Geometry: final body of the model. Coordinates: model frame, mm. Face numbers are marked on the shaded views. A direction names the side the tool comes from. Round coordinates to 2 decimals unless told otherwise and drop trailing zeros. Loops run counter-clockwise (first coordinate to the right, second up) from the corner with the lowest first, then second, coordinate; pieces in that order, holes last. Notation, with made-up numbers: M -12,31.5 L 3,31.5 A23 ccw 3,63.5 Z; hole C 82.5,22 d11. An arc over 180 degrees is marked long. Return JSON: item names as keys, results as strings.
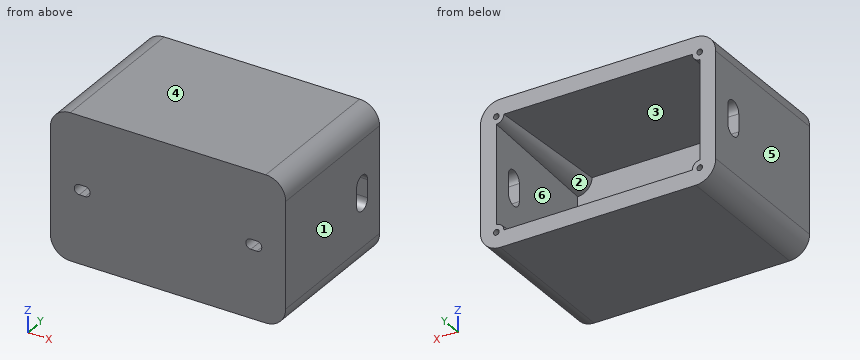
from build123d import *

# Parameters (mm, degrees)
SKETCH1_W                     = 118
SKETCH1_H                     = 73
BOSS_EXTRUDE1_DEPTH           = 75
SKETCH3_W                     = 102
SKETCH3_H                     = 57
CUT_EXTRUDE2_DEPTH            = 65
FILLET1_R                     = 10
CUT_EXTRUDE3_DEPTH            = 103.167754208
SKETCH5_R                     = 7.171572875
BOSS_EXTRUDE2_DEPTH           = 65
BOSS_EXTRUDE2_DRAFT           = 3
BOSS_EXTRUDE2_PROFILE_2_DEPTH = 65
BOSS_EXTRUDE2_PROFILE_2_DRAFT = 3
BOSS_EXTRUDE2_PROFILE_3_DEPTH = 65
BOSS_EXTRUDE2_PROFILE_3_DRAFT = 3
BOSS_EXTRUDE2_PROFILE_4_DEPTH = 65
BOSS_EXTRUDE2_PROFILE_4_DRAFT = 3
SKETCH9_R                     = 1.4
CUT_EXTRUDE6_DEPTH            = 5
CUT_EXTRUDE7_DEPTH            = 10000


with BuildPart() as part:
    # Sketch1 → Boss-Extrude1 (new body)
    with BuildSketch(Plane(origin=(0, 0, 0), x_dir=(1, 0, 0), z_dir=(0, 1, 0))):
        Rectangle(SKETCH1_W, SKETCH1_H)
    extrude(amount=BOSS_EXTRUDE1_DEPTH)

    # Sketch3 → Cut-Extrude2 (cut)
    with BuildSketch(Plane(origin=(0, 75, 0), x_dir=(1, 0, 0), z_dir=(0, 1, 0))):
        Rectangle(SKETCH3_W, SKETCH3_H)
    extrude(amount=-CUT_EXTRUDE2_DEPTH, mode=Mode.SUBTRACT)

    # Fillet1
    fillet1_edges = [part.edges().sort_by_distance(p)[0] for p in [
        (-59, 37.5, -36.5),
        (59, 37.5, -36.5),
        (59, 37.5, 36.5),
        (-59, 37.5, 36.5),
    ]]
    fillet(fillet1_edges, radius=FILLET1_R)

    # Sketch4 → Cut-Extrude3 (cut, through all)
    with BuildSketch(Plane.XZ):
        with BuildLine():
            Line((-44.5, -2.5), (-41.5, -2.5))
            ThreePointArc((-41.5, -2.5), (-39, 0), (-41.5, 2.5))
            Line((-41.5, 2.5), (-44.5, 2.5))
            ThreePointArc((-44.5, 2.5), (-47, 0), (-44.5, -2.5))
        make_face()
        with BuildLine():
            ThreePointArc((41.5, -2.5), (39, 0), (41.5, 2.5))
            Line((41.5, 2.5), (44.5, 2.5))
            ThreePointArc((44.5, 2.5), (47, 0), (44.5, -2.5))
            Line((44.5, -2.5), (41.5, -2.5))
        make_face()
    extrude(amount=-CUT_EXTRUDE3_DEPTH, mode=Mode.SUBTRACT)


with BuildPart() as boss_extrude2_tool:
    # Sketch5 → Boss-Extrude2 (with draft: the straight prism first)
    with BuildSketch(Plane(origin=(0, 10, 0), x_dir=(1, 0, 0), z_dir=(0, 1, 0))):
        with Locations((-51, 28.5)):
            Circle(SKETCH5_R)
    extrude(amount=BOSS_EXTRUDE2_DEPTH)
    # Boss-Extrude2: the draft: its side faces are tilted about the plane it starts from
    boss_extrude2_sides = [boss_extrude2_tool.faces().sort_by_distance(p)[0] for p in [
        (-58.171572875, 42.5, -28.5),
    ]]
    draft(boss_extrude2_sides, Plane(origin=(0, 10, 0), x_dir=(1, 0, 0), z_dir=(0, 1, 0)), BOSS_EXTRUDE2_DRAFT)


with BuildPart() as part_1:
    add(part.part)

    # Boss-Extrude2: add boss_extrude2_tool
    add(boss_extrude2_tool.part)


with BuildPart() as boss_extrude2_profile_2_tool:
    # Sketch5 → Boss-Extrude2 profile 2 (with draft: the straight prism first)
    with BuildSketch(Plane(origin=(0, 10, 0), x_dir=(1, 0, 0), z_dir=(0, 1, 0))):
        with Locations((51, 28.5)):
            Circle(SKETCH5_R)
    extrude(amount=BOSS_EXTRUDE2_PROFILE_2_DEPTH)
    # Boss-Extrude2 profile 2: the draft: its side faces are tilted about the plane it starts from
    boss_extrude2_profile_2_sides = [boss_extrude2_profile_2_tool.faces().sort_by_distance(p)[0] for p in [
        (43.828427125, 42.5, -28.5),
    ]]
    draft(boss_extrude2_profile_2_sides, Plane(origin=(0, 10, 0), x_dir=(1, 0, 0), z_dir=(0, 1, 0)), BOSS_EXTRUDE2_PROFILE_2_DRAFT)


with BuildPart() as part_2:
    add(part_1.part)

    # Boss-Extrude2 profile 2: add boss_extrude2_profile_2_tool
    add(boss_extrude2_profile_2_tool.part)


with BuildPart() as boss_extrude2_profile_3_tool:
    # Sketch5 → Boss-Extrude2 profile 3 (with draft: the straight prism first)
    with BuildSketch(Plane(origin=(0, 10, 0), x_dir=(1, 0, 0), z_dir=(0, 1, 0))):
        with Locations((51, -28.5)):
            Circle(SKETCH5_R)
    extrude(amount=BOSS_EXTRUDE2_PROFILE_3_DEPTH)
    # Boss-Extrude2 profile 3: the draft: its side faces are tilted about the plane it starts from
    boss_extrude2_profile_3_sides = [boss_extrude2_profile_3_tool.faces().sort_by_distance(p)[0] for p in [
        (43.828427125, 42.5, 28.5),
    ]]
    draft(boss_extrude2_profile_3_sides, Plane(origin=(0, 10, 0), x_dir=(1, 0, 0), z_dir=(0, 1, 0)), BOSS_EXTRUDE2_PROFILE_3_DRAFT)


with BuildPart() as part_3:
    add(part_2.part)

    # Boss-Extrude2 profile 3: add boss_extrude2_profile_3_tool
    add(boss_extrude2_profile_3_tool.part)


with BuildPart() as boss_extrude2_profile_4_tool:
    # Sketch5 → Boss-Extrude2 profile 4 (with draft: the straight prism first)
    with BuildSketch(Plane(origin=(0, 10, 0), x_dir=(1, 0, 0), z_dir=(0, 1, 0))):
        with Locations((-51, -28.5)):
            Circle(SKETCH5_R)
    extrude(amount=BOSS_EXTRUDE2_PROFILE_4_DEPTH)
    # Boss-Extrude2 profile 4: the draft: its side faces are tilted about the plane it starts from
    boss_extrude2_profile_4_sides = [boss_extrude2_profile_4_tool.faces().sort_by_distance(p)[0] for p in [
        (-58.171572875, 42.5, 28.5),
    ]]
    draft(boss_extrude2_profile_4_sides, Plane(origin=(0, 10, 0), x_dir=(1, 0, 0), z_dir=(0, 1, 0)), BOSS_EXTRUDE2_PROFILE_4_DRAFT)


with BuildPart() as part_4:
    add(part_3.part)

    # Boss-Extrude2 profile 4: add boss_extrude2_profile_4_tool
    add(boss_extrude2_profile_4_tool.part)

    # Sketch9 → Cut-Extrude6 (cut)
    with BuildSketch(Plane(origin=(0, 75, 0), x_dir=(1, 0, 0), z_dir=(0, 1, 0))):
        with Locations(Location((-51, 28.5, 0), (0, 0, 270))):
            Circle(SKETCH9_R)
        with Locations(Location((51, 28.5, 0), (0, 0, 90))):
            Circle(SKETCH9_R)
        with Locations(Location((51, -28.5, 0), (0, 0, 270))):
            Circle(SKETCH9_R)
        with Locations(Location((-51, -28.5, 0), (0, 0, 90))):
            Circle(SKETCH9_R)
    extrude(amount=-CUT_EXTRUDE6_DEPTH, mode=Mode.SUBTRACT)

    # Sketch13 → Cut-Extrude7 (cut)
    with BuildSketch(Plane.ZY.offset(59)):
        with BuildLine():
            Line((-4.178843904, 65.399928421), (4.670472599, 65.399928421))
            ThreePointArc((4.670472599, 65.399928421), (9.07040102, 61), (4.670472599, 56.600071579))
            Line((4.670472599, 56.600071579), (-4.178843904, 56.600071579))
            ThreePointArc((-4.178843904, 56.600071579), (-8.578772325, 61), (-4.178843904, 65.399928421))
        make_face()
    extrude(amount=-CUT_EXTRUDE7_DEPTH, mode=Mode.SUBTRACT)


solid = part_4.part
Q1. Section query C-C (z = 16). Output: boundary loops of the cut face in (x, y), plus the area to 3 significant figures.
Determined:
{"outline": "M -59,0 L 59,0 L 59,75 L 51,75 L 51,10 L -51,10 L -51,75 L -59,75 Z", "area": "2,220 mm^2"}
Q2. Pull-direction query (X, two-part tool) for the marked faces 1, 2, 3 and 4; classes: pulls with the +X half, pulls with the -X half, needs draft (parallel to the pull), parting line crosses it, or undercut.
Determined:
{"face 1": "pulls with the +X half", "face 2": "undercut", "face 3": "undercut", "face 4": "needs draft"}
Q3. Reachability of the marked faces 5 and 6 from +Z, -Z, +X, -X, +Y, -Y: full face, straight path, thin tool, end or side. Return the list, or none.
Determined:
{"face 5": "+Z, -Z, -X, +Y, -Y", "face 6": "+Y"}
Q4. Pin query (flat end, axial travel): pin 1 (2 mm diameter, centred on x = 51, z = 28.5, fed in from +Y); pin 2 (6 mm diameter, centred on x = 7, z = -19, fed in from +Y). Return the tip coordinate at first contact, or that it passes through.
Determined:
{"pin 1": "stops at y = 70", "pin 2": "stops at y = 10"}
Q5. Section query B-B (x = 4.5). Output: boundary loops of the cut face in (y, z).
Determined:
{"outline": "M 0,-36.5 L 75,-36.5 L 75,-28.5 L 10,-28.5 L 10,28.5 L 75,28.5 L 75,36.5 L 0,36.5 Z"}
Q6. Material intervals for L1, parallel to Z at x = 6.5, y = 52.5; L2, parallel to X at y = 69, z = 4.5; L3, parallel to Y at x = 2, z = -16.5, sorted ascending.
Determined:
{"L1": "z = -36.5 to -28.5, 28.5 to 36.5", "L2": "x = -59 to -51, 51 to 59", "L3": "y = 0 to 10"}
Q7. Section query D-D (y = 28.5). Output: boundary loops of the cut face in (x, z), plus the area to 4 significant figures.
Determined:
{"outline": "M -59,-26.5 A10 ccw -49,-36.5 L 49,-36.5 A10 ccw 59,-26.5 L 59,26.5 A10 ccw 49,36.5 L -49,36.5 A10 ccw -59,26.5 Z; hole M -51,-22.3 A6.2 cw -44.8,-28.5 L 44.8,-28.5 A6.2 cw 51,-22.3 L 51,22.3 A6.2 cw 44.8,28.5 L -44.8,28.5 A6.2 cw -51,22.3 Z", "area": "2,835 mm^2"}
Q8. Section query A-A (y = 61). Output: boundary loops of the cut face in (x, z), plus the area to 3 significant figures.
Determined:
{"outline": "M -59,-26.5 A10 ccw -49,-36.5 L 49,-36.5 A10 ccw 59,-26.5 L 59,-8.58 L 51,-8.58 L 51,-24 A4.5 ccw 46.5,-28.5 L -46.5,-28.5 A4.5 ccw -51,-24 L -51,-8.58 L -59,-8.58 Z; M -59,9.07 L -51,9.07 L -51,24 A4.5 ccw -46.5,28.5 L 46.5,28.5 A4.5 ccw 51,24 L 51,9.07 L 59,9.07 L 59,26.5 A10 ccw 49,36.5 L -49,36.5 A10 ccw -59,26.5 Z", "area": "2,500 mm^2"}
